For this review, take the finished solid that the model builds, in its own axes (mm). Coordinates: 2 decimals unless noted, no trailing zeros. Loops run counter-clockwise (first coordinate to the right, second up) from the corner with the lowest first, then second, coordinate; pieces in that order, holes last. Notation, with made-up numbers: (37.25, 42.5) -> (91.25, 42.5) arc R23 ccw to (91.25, 67.5) -> close; hole circle Ø8 at (5, 41.25). An arc over 180 degrees is marked (long way). Answer in a Markdown table with one row per item.
from build123d import *

# Parameters (mm, degrees)
SKETCH1_R           = 3.5
BOSS_EXTRUDE1_DEPTH = 1.6
SKETCH2_R           = 1.25
CUT_EXTRUDE1_DEPTH  = 2.6
CHAMFER1_SIZE       = 0.1


with BuildPart() as part:
    # Sketch1 → Boss-Extrude1 (new body)
    with BuildSketch(Plane.XY):
        Circle(SKETCH1_R)
    extrude(amount=-BOSS_EXTRUDE1_DEPTH)

    # Sketch2 → Cut-Extrude1 (cut, through all)
    with BuildSketch(Plane.XY):
        Circle(SKETCH2_R)
    extrude(amount=-CUT_EXTRUDE1_DEPTH, mode=Mode.SUBTRACT)

    # Chamfer1
    chamfer1_edges = [part.edges().sort_by_distance(p)[0] for p in [
        (-1.25, 0, -1.6),
        (-1.25, 0, 0),
    ]]
    chamfer(chamfer1_edges, length=CHAMFER1_SIZE)


solid = part.part
Item 1: Take a section at C-C, the plane z = -1.25. State the section outline as (x, y) points.
Worked answers:
| item | result |
|---|---|
| outline | circle Ø7 at (0, 0); hole circle Ø2.5 at (0, 0) |
Item 2: For L1, parallel to Y at x = 0, z = -1; L2, parallel to X at y = 0.25, z = -0.4; L3, parallel to Y at x = -0.5, z = -0.3, list the stretches that pass through material, from the lowest coordinate up.
Worked answers:
| item | result |
|---|---|
| L1 | -3.5 to -1.25, 1.25 to 3.5 |
| L2 | -3.49 to -1.22, 1.22 to 3.49 |
| L3 | -3.46 to -1.15, 1.15 to 3.46 |
Item 3: Take a section at D-D, the plane y = -1.5. State the section outline as (x, z) points, and give its area (3 significant figures).
Worked answers:
| item | result |
|---|---|
| outline | (-3.16, -1.6) -> (3.16, -1.6) -> (3.16, 0) -> (-3.16, 0) -> close |
| area | 10.1 mm² |
Item 4: The part is to be moulded in two halves that separate along X. For faces 1 (the cylindrical face through (-0.27, -1.22, -0.79)), 2 (the cylindrical face through (3.233, -1.341, -0.789)), 3 (the flat face through (0, -2, 0)), say which applies: +X half, -X half, draft (parallel to the pull), parting line (faces both ways), or undercut.
Worked answers:
| item | result |
|---|---|
| face 1 | undercut |
| face 2 | parting line |
| face 3 | draft |
Item 5: Insertion check: pin 1 (3 mm diameter, centred on x = 1, y = 2, fed in from +Z); pin 2 (1.5 mm diameter, centred on x = 0, y = 0, fed in from +Z). Each pin has a flat end and moves straight along its axis. Give the tip position at first contact, or say it passes through.
Worked answers:
| item | result |
|---|---|
| pin 1 | z = 0 |
| pin 2 | through |
Item 6: Take a section at A-A, the plane y = 0. State the section outline as (x, z) points, and give its area (3 significant figures).
Worked answers:
| item | result |
|---|---|
| outline | (-3.5, -1.6) -> (-1.35, -1.6) -> (-1.25, -1.5) -> (-1.25, -0.1) -> (-1.35, 0) -> (-3.5, 0) -> close; (1.25, -1.5) -> (1.35, -1.6) -> (3.5, -1.6) -> (3.5, 0) -> (1.35, 0) -> (1.25, -0.1) -> close |
| area | 7.18 mm² |
